For this review, take the finished solid that the model builds, in its own axes (mm). A direction names the side the tool comes from. Give positions to 0.01 mm unless a question says otherwise; leave off trailing zeros. Loops run counter-clockwise (first coordinate to the right, second up) from the corner with the lowest first, then second, coordinate; pieces in that order, holes last. Notation, with made-up numbers: (-0.75, 21.5) - (55.25, 21.5) arc R24 cw to (55.25, 59.5) - close; hole circle Ø9 at (-9.5, 18.25). An arc over 180 degrees is marked (long way). Use CSV: the item, a comma, the result in double quotes. Start each with the question number.
1. Mouldability with a two-part tool opening along X and no side actions: class faces 3 (the cylindrical face through (-18.897, 3.131, -14.49)), 4 (the cylindrical face through (3.186, 3.219, 0.165)), 5 (the flat face through (5, 6.35, 5)), 6 (the cylindrical face through (-4.21, 3.22, 3.83)) as pulls with the +X half, pulls with the -X half, needs draft (parallel to the pull), parting line crosses it, or undercut.
2. Take a section at B-B on x = 8.89. Give the boundary of the cut face in (y, z).
3. Take a section at C-C on y = 5.25. State how many separate pieces and enclosed holes the cut face has, plus the area to 3 significant figures.
4. Wall thickness on line 1 (Z direction, x = 6.5, y = 2.25); line 2 (X direction, y = 3.75, z = -17.5); line 3 (Z direction, x = -18, y = 2.5): over which ranges is each line inside the solid? List them lowest first.
5. Take a section at A-A on z = 18.5. Give the boundary of the cut face in (x, y).
6. For pin 1 (5 mm diameter, centred on x = -1.5, z = 16.5, fed in from -Y); pin 2 (4 mm diameter, centred on x = 0, z = 17.46, fed in from -Y); pin 3 (4 mm diameter, centred on x = 0, z = -8.89, fed in from -Y); pin 4 (3 mm diameter, centred on x = -9.5, y = 4.5, fed in from -Z), all flat-tipped, find the tip position at first contact; note any pin that passes through.
7. For faces 1 (the cylindrical face through (0.17, 3.22, -7.63)), 2 (the cylindrical face through (22.22, 1.69, -0.21)), list the 3-axis set-ups (+Z, -Z, +X, -X, +Y, -Y) from which the entire face can be reached by the end or side of a thin tool; tool diameter is ignored.
```python
from build123d import *

# Parameters (mm, degrees)
SKETCH1_R                                           = 50.8
BOSS_EXTRUDE1_DEPTH                                 = 25.4
SKETCH2_R                                           = 69.85
SKETCH2_R_2                                         = 50.8
BOSS_EXTRUDE2_DEPTH                                 = 12.7
SKETCH3_R                                           = 49.53
SKETCH3_R_2                                         = 47.625
CUT_EXTRUDE1_DEPTH                                  = 1.1176
CUT_EXTRUDE2_REACH                                  = 27.4
SKETCH4_R                                           = 3.175
SKETCH5_R                                           = 11.43
CUT_EXTRUDE3_DEPTH                                  = 19.05
CUT_EXTRUDE4_REACH                                  = 8.35
SKETCH6_R                                           = 1.5875
SKETCH42_OUTSIDE_W                                  = 181.538
SKETCH42_OUTSIDE_H                                  = 181.538
SKETCH42_OUTSIDE_R                                  = 23.8125
CUT_EXTRUDE9_DEPTH                                  = 30.48
SKETCH43_R                                          = 20.6375
CUT_EXTRUDE10_DEPTH                                 = 19.05
CBORE_FOR_10_BINDING_HEAD_MACHINE_SCREW_D           = 4.9784
CBORE_FOR_10_BINDING_HEAD_MACHINE_SCREW_CBORE_D     = 9.525
CBORE_FOR_10_BINDING_HEAD_MACHINE_SCREW_CBORE_DEPTH = 3.429
SKETCH52_R                                          = 23.8125
CUT_EXTRUDE11_DEPTH                                 = 19.05
SKETCH54_R                                          = 1.27
CUT_EXTRUDE12_DEPTH                                 = 6.35
CIRPATTERN1_COUNT                                   = 8
SKETCH55_R                                          = 1.27
CUT_EXTRUDE13_DEPTH                                 = 6.35
CIRPATTERN2_COUNT                                   = 8


with BuildPart() as part:
    # Sketch1 → Boss-Extrude1 (new body)
    with BuildSketch(Plane(origin=(0, 0, 0), x_dir=(1, 0, 0), z_dir=(0, 1, 0))):
        Circle(SKETCH1_R)
    extrude(amount=BOSS_EXTRUDE1_DEPTH)

    # Sketch2 → Boss-Extrude2 (add)
    with BuildSketch(Plane.XZ):
        Circle(SKETCH2_R)
        Circle(SKETCH2_R_2, mode=Mode.SUBTRACT)
    extrude(amount=-BOSS_EXTRUDE2_DEPTH)

    # Sketch3 → Cut-Extrude1 (cut)
    with BuildSketch(Plane.XZ):
        Circle(SKETCH3_R)
        Circle(SKETCH3_R_2, mode=Mode.SUBTRACT)
    extrude(amount=-CUT_EXTRUDE1_DEPTH, mode=Mode.SUBTRACT)

    # Sketch4 → Cut-Extrude2 (cut, up to next)
    with BuildSketch(Plane.XZ, mode=Mode.PRIVATE) as cut_extrude2_sk1:
        with Locations((0, -59.9186)):
            Circle(SKETCH4_R)
    cut_extrude2_tool1 = extrude(cut_extrude2_sk1.sketch, amount=-CUT_EXTRUDE2_REACH, mode=Mode.PRIVATE) & part.part
    add(cut_extrude2_tool1.solids().sort_by_distance((0, 0, -59.9186))[0], mode=Mode.SUBTRACT)
    # Sketch4 → Cut-Extrude2 (cut, up to next)
    with BuildSketch(Plane.XZ, mode=Mode.PRIVATE) as cut_extrude2_sk2:
        with Locations((-42.368848379, -42.368848379)):
            Circle(SKETCH4_R)
    cut_extrude2_tool2 = extrude(cut_extrude2_sk2.sketch, amount=-CUT_EXTRUDE2_REACH, mode=Mode.PRIVATE) & part.part
    add(cut_extrude2_tool2.solids().sort_by_distance((-42.368848, 0, -42.368848))[0], mode=Mode.SUBTRACT)
    # Sketch4 → Cut-Extrude2 (cut, up to next)
    with BuildSketch(Plane.XZ, mode=Mode.PRIVATE) as cut_extrude2_sk3:
        with Locations((-59.9186, 0)):
            Circle(SKETCH4_R)
    cut_extrude2_tool3 = extrude(cut_extrude2_sk3.sketch, amount=-CUT_EXTRUDE2_REACH, mode=Mode.PRIVATE) & part.part
    add(cut_extrude2_tool3.solids().sort_by_distance((-59.9186, 0, 0))[0], mode=Mode.SUBTRACT)
    # Sketch4 → Cut-Extrude2 (cut, up to next)
    with BuildSketch(Plane.XZ, mode=Mode.PRIVATE) as cut_extrude2_sk4:
        with Locations((-42.368848379, 42.368848379)):
            Circle(SKETCH4_R)
    cut_extrude2_tool4 = extrude(cut_extrude2_sk4.sketch, amount=-CUT_EXTRUDE2_REACH, mode=Mode.PRIVATE) & part.part
    add(cut_extrude2_tool4.solids().sort_by_distance((-42.368848, 0, 42.368848))[0], mode=Mode.SUBTRACT)
    # Sketch4 → Cut-Extrude2 (cut, up to next)
    with BuildSketch(Plane.XZ, mode=Mode.PRIVATE) as cut_extrude2_sk5:
        with Locations((0, 59.9186)):
            Circle(SKETCH4_R)
    cut_extrude2_tool5 = extrude(cut_extrude2_sk5.sketch, amount=-CUT_EXTRUDE2_REACH, mode=Mode.PRIVATE) & part.part
    add(cut_extrude2_tool5.solids().sort_by_distance((0, 0, 59.9186))[0], mode=Mode.SUBTRACT)
    # Sketch4 → Cut-Extrude2 (cut, up to next)
    with BuildSketch(Plane.XZ, mode=Mode.PRIVATE) as cut_extrude2_sk6:
        with Locations((42.368848379, 42.368848379)):
            Circle(SKETCH4_R)
    cut_extrude2_tool6 = extrude(cut_extrude2_sk6.sketch, amount=-CUT_EXTRUDE2_REACH, mode=Mode.PRIVATE) & part.part
    add(cut_extrude2_tool6.solids().sort_by_distance((42.368848, 0, 42.368848))[0], mode=Mode.SUBTRACT)
    # Sketch4 → Cut-Extrude2 (cut, up to next)
    with BuildSketch(Plane.XZ, mode=Mode.PRIVATE) as cut_extrude2_sk7:
        with Locations((59.9186, 0)):
            Circle(SKETCH4_R)
    cut_extrude2_tool7 = extrude(cut_extrude2_sk7.sketch, amount=-CUT_EXTRUDE2_REACH, mode=Mode.PRIVATE) & part.part
    add(cut_extrude2_tool7.solids().sort_by_distance((59.9186, 0, 0))[0], mode=Mode.SUBTRACT)
    # Sketch4 → Cut-Extrude2 (cut, up to next)
    with BuildSketch(Plane.XZ, mode=Mode.PRIVATE) as cut_extrude2_sk8:
        with Locations((42.368848379, -42.368848379)):
            Circle(SKETCH4_R)
    cut_extrude2_tool8 = extrude(cut_extrude2_sk8.sketch, amount=-CUT_EXTRUDE2_REACH, mode=Mode.PRIVATE) & part.part
    add(cut_extrude2_tool8.solids().sort_by_distance((42.368848, 0, -42.368848))[0], mode=Mode.SUBTRACT)

    # Sketch5 → Cut-Extrude3 (cut)
    with BuildSketch(Plane(origin=(0, 25.4, 0), x_dir=(1, 0, 0), z_dir=(0, 1, 0))):
        Circle(SKETCH5_R)
    extrude(amount=-CUT_EXTRUDE3_DEPTH, mode=Mode.SUBTRACT)

    # Sketch6 → Cut-Extrude4 (cut, up to next)
    with BuildSketch(Plane(origin=(0, 6.35, 0), x_dir=(1, 0, 0), z_dir=(0, 1, 0)), mode=Mode.PRIVATE) as cut_extrude4_sk1:
        Circle(SKETCH6_R)
    cut_extrude4_tool1 = extrude(cut_extrude4_sk1.sketch, amount=-CUT_EXTRUDE4_REACH, mode=Mode.PRIVATE) & part.part
    add(cut_extrude4_tool1.solids().sort_by_distance((0, 6.35, 0))[0], mode=Mode.SUBTRACT)

    # Sketch42 outside → Cut-Extrude9 (cut)
    with BuildSketch(Plane.XZ):
        Rectangle(SKETCH42_OUTSIDE_W, SKETCH42_OUTSIDE_H)
        Circle(SKETCH42_OUTSIDE_R, mode=Mode.SUBTRACT)
    extrude(amount=-CUT_EXTRUDE9_DEPTH, mode=Mode.SUBTRACT)

    # Sketch43 → Cut-Extrude10 (cut)
    with BuildSketch(Plane(origin=(0, 25.4, 0), x_dir=(1, 0, 0), z_dir=(0, 1, 0))):
        Circle(SKETCH43_R)
    extrude(amount=-CUT_EXTRUDE10_DEPTH, mode=Mode.SUBTRACT)

    # CBORE for #10 Binding Head Machine Screw1 (through all)
    with Locations(Plane(origin=(0, 0, 0), x_dir=(-1, 0, 0), z_dir=(0, -1, 0))):
        with Locations((0, -17.4625), (-17.4625, 0), (17.4625, 0), (0, 17.4625)):
            CounterBoreHole(CBORE_FOR_10_BINDING_HEAD_MACHINE_SCREW_D / 2, CBORE_FOR_10_BINDING_HEAD_MACHINE_SCREW_CBORE_D / 2, CBORE_FOR_10_BINDING_HEAD_MACHINE_SCREW_CBORE_DEPTH)

    # Sketch52 → Cut-Extrude11 (cut)
    with BuildSketch(Plane(origin=(0, 25.4, 0), x_dir=(1, 0, 0), z_dir=(0, 1, 0))):
        Circle(SKETCH52_R)
    extrude(amount=-CUT_EXTRUDE11_DEPTH, mode=Mode.SUBTRACT)

    # Sketch54 → Cut-Extrude12 (cut)
    with BuildSketch(Plane(origin=(0, 6.35, 0), x_dir=(1, 0, 0), z_dir=(0, 1, 0))):
        with Locations((0, -4.445)):
            Circle(SKETCH54_R)
    cut_extrude12 = extrude(amount=-CUT_EXTRUDE12_DEPTH, mode=Mode.SUBTRACT)

    # CirPattern1: Cut-Extrude12 ×8 about axis
    cirpattern1_axis = Axis((0, 0, 0), (0, 1, 0))
    for i in range(1, CIRPATTERN1_COUNT):
        add(cut_extrude12.rotate(cirpattern1_axis, i * 360 / CIRPATTERN1_COUNT), mode=Mode.SUBTRACT)

    # Sketch55 → Cut-Extrude13 (cut)
    with BuildSketch(Plane(origin=(0, 6.35, 0), x_dir=(1, 0, 0), z_dir=(0, 1, 0))):
        with Locations((0, -8.89)):
            Circle(SKETCH55_R)
    cut_extrude13 = extrude(amount=-CUT_EXTRUDE13_DEPTH, mode=Mode.SUBTRACT)

    # CirPattern2: Cut-Extrude13 ×8 about axis
    cirpattern2_axis = Axis((0, 0, 0), (0, 1, 0))
    for i in range(1, CIRPATTERN2_COUNT):
        add(cut_extrude13.rotate(cirpattern2_axis, i * 360 / CIRPATTERN2_COUNT), mode=Mode.SUBTRACT)


solid = part.part
```
Check result:
1,face 3,"parting line crosses it"
1,face 4,"undercut"
1,face 5,"needs draft"
1,face 6,"undercut"
2,outline,"(0, -22.09) - (6.35, -22.09) - (6.35, -1.27) - (0, -1.27) - close; (0, 1.27) - (6.35, 1.27) - (6.35, 22.09) - (0, 22.09) - close"
3,separate pieces,"1"
3,enclosed holes,"21"
3,area,"1,610 mm²"
4,line 1,"z = -22.91 to -7.54, -5.03 to 5.03, 7.54 to 22.91"
4,line 2,"x = -16.15 to -2.49, 2.49 to 16.15"
4,line 3,"z = -15.59 to -4.73, 4.73 to 15.59"
5,outline,"(-14.99, 0) - (-4.65, 0) - (-4.65, 3.43) - (-2.26, 3.43) - (-2.26, 6.35) - (-14.99, 6.35) - close; (2.26, 3.43) - (4.65, 3.43) - (4.65, 0) - (14.99, 0) - (14.99, 6.35) - (2.26, 6.35) - close"
6,pin 1,"stops at y = 3.43"
6,pin 2,"passes through"
6,pin 3,"stops at y = 0"
6,pin 4,"stops at z = -22.43"
7,face 1,"+Y, -Y"
7,face 2,"-Y"
